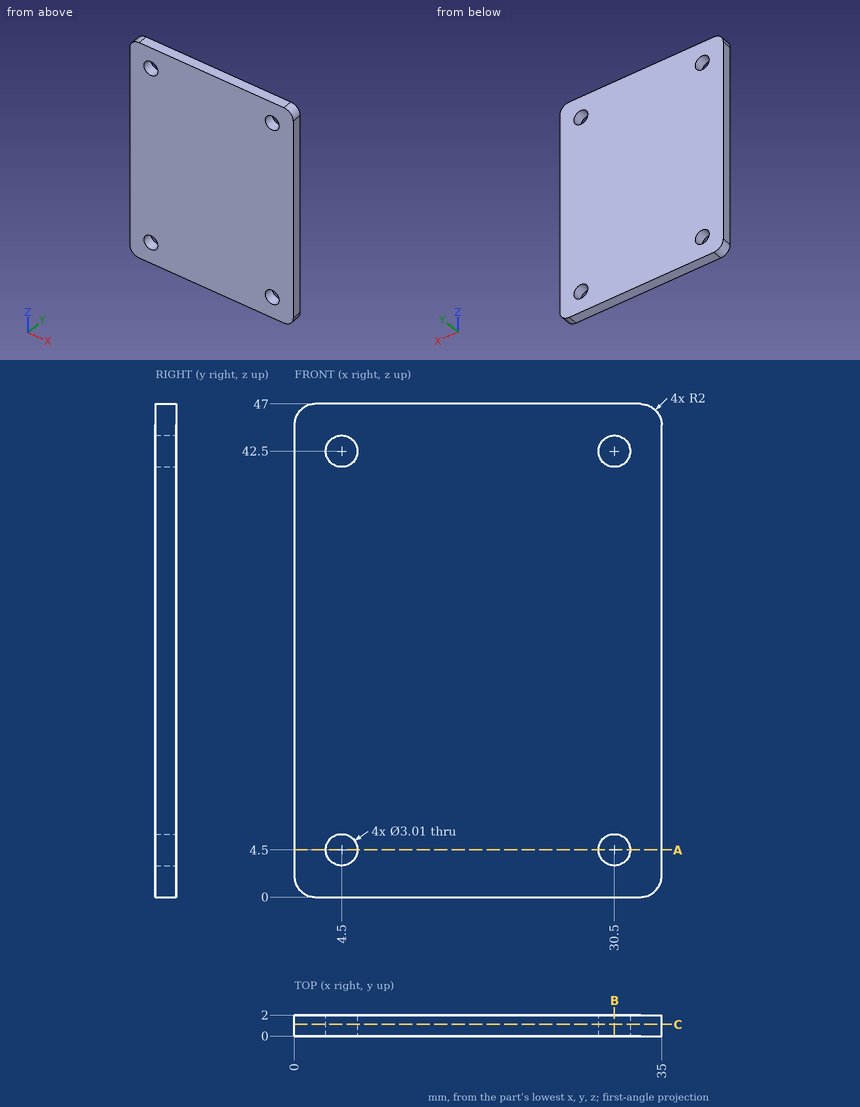
Answer from the drawing. Dimensions are ordinates in mm from the lowest x, y and z of the part. Give positions to 0.01 mm unless a question says otherwise; leave off trailing zeros. Order: outer loops, then holes, each group sorted by start corner. A loop starts at its lowest first (then second) coordinate and runs counter-clockwise, first axis right, second up.
(1) Find section A-A (z = 4.5). Give the vertices of the cut face in (x, y) (3 decimals), plus the area to 3 significant figures.
(2) Find section B-B (x = 30.5). Give the vertices of the cut face in (y, z) (3 decimals).
(3) Straight lines are drawn through the part: L1, parallel to Z at x = 4.5, y = 0.4 (3 decimals); L2, parallel to X at y = 1.55, z = 4.5 (3 decimals); L3, parallel to Z at x = 5.5, y = 0.35. For each, find the intervals that lie inside material, in ascending order.
(4) Given pin 1 (1.8 mm diameter, centred on x = 4.5, z = 42.5, fed in from -Y), flat-ended and moving along its own axis, determine where the tip first touches the part or whether it passes through.
(5) Find section C-C (y = 1.1). Give the vertices of the cut face in (x, z) (3 decimals).
Result sheet:
1. outline: (0, 0) - (2.995, 0) - (2.995, 2) - (0, 2) - close; (6.005, 0) - (28.995, 0) - (28.995, 2) - (6.005, 2) - close; (32.005, 0) - (35, 0) - (35, 2) - (32.005, 2) - close
1. area: 58.0 mm2
2. outline: (0, 0) - (2, 0) - (2, 2.995) - (0, 2.995) - close; (0, 6.005) - (2, 6.005) - (2, 40.995) - (0, 40.995) - close; (0, 44.005) - (2, 44.005) - (2, 47) - (0, 47) - close
3. L1: z = 0 to 2.995, 6.005 to 40.995, 44.005 to 47
3. L2: x = 0 to 2.995, 6.005 to 28.995, 32.005 to 35
3. L3: z = 0 to 3.38, 5.62 to 41.38, 43.62 to 47
4. pin 1: passes through
5. outline: (0, 2) arc R2 ccw to (2, 0) - (33, 0) arc R2 ccw to (35, 2) - (35, 45) arc R2 ccw to (33, 47) - (2, 47) arc R2 ccw to (0, 45) - close; hole circle Ø3.01 at (4.5, 4.5); hole circle Ø3.01 at (4.5, 42.5); hole circle Ø3.01 at (30.5, 4.5); hole circle Ø3.01 at (30.5, 42.5)
